The model under review builds one solid part; all positions refer to its coordinate system, in mm. A direction names the side the tool comes from. Coordinates: 2 decimals unless noted, no trailing zeros. Loops run counter-clockwise (first coordinate to the right, second up) from the corner with the lowest first, then second, coordinate; pieces in that order, holes last. Notation, with made-up numbers: M 33,44.5 L 41,44.5 A22 ccw 41,73.5 Z; hole C -5,83.25 d6. An arc over 180 degrees is marked long. Use CSV: the item, a comma, the result in double quotes. Start each with the question number.
1. Tool access review of faces 1 (the flat face through (-16, 6, 29.5)), 2 (the flat face through (-0.14, 3.72, -30.36)), 3 (the flat face through (-0.1, 8.5, 31)), 4 (the flat face through (21.25, 2, 0)), 5 (the flat face through (-21.25, 7, 0)): name each direction out of +Z, -Z, +X, -X, +Y, -Y from which nothing blocks a thin tool from reaching the whole face with its end or side.
2. Add section C-C, the plane x = -14.5. Write out the cut boundary in (y, z), then the cut area to 3 significant figures.
3. Add section B-B, the plane y = 5.25. Write out the cut boundary in (x, z), then the cut area to 3 significant figures.
4. Clearance check with flat-ended pins moving along their axes: P1, Ø2, axis at x = -4.5, y = 7, coming from the -Z side; P2, Ø5, axis at x = 13.5, y = 6.5, coming from the -Z side; P3, Ø0.5, axis at y = 7, z = -30, coming from the -X side. State where each tip first meets the part, or that it passes through.
5. Add section D-D, the plane z = -8.5. Write out the cut boundary in (x, y).
6. Draft analysis for pull direction Y (two halves, no side actions). For faces 6 (the flat face through (0, 0, 0)), 7 (the flat face through (10, 5, -30)), 8 (the flat face through (0, 1, -32.5)), state which applies: +Y half, -Y half, draft (parallel to the pull), parting line (faces both ways), or undercut.
7. For L1, parallel to Y at x = -1, z = 7; L2, parallel to Z at x = 19, y = 7; L3, parallel to X at y = 8.5, z = -30, list the stretches that pass through material, from the lowest coordinate up.
8. Add section A-A, the plane x = 7.5. Write out the cut boundary in (y, z), then the cut area to 3 significant figures.
from build123d import *

# Parameters (mm, degrees)
SKETCH1_W            = 46.5
SKETCH1_H            = 65
BOSS_EXTRUDE1_DEPTH  = 1.5
FILLET1_R            = 3
SKETCH2_W            = 20
SKETCH2_H            = 1.5
BOSS_EXTRUDE2_DEPTH  = 8
CUT_EXTRUDE1_DEPTH   = 24
BOSS_EXTRUDE5_DEPTH  = 20
FILLET4_R            = 0.5
FILLET4_OF_MIRROR1_R = 0.5
BOSS_EXTRUDE6_DEPTH  = 1.5
BOSS_EXTRUDE7_DEPTH  = 0.5
BOSS_EXTRUDE8_START  = -9
BOSS_EXTRUDE8_DEPTH  = 9


with BuildPart() as part:
    # Sketch1 → Boss-Extrude1 (new body)
    with BuildSketch(Plane(origin=(0, 0, 0), x_dir=(1, 0, 0), z_dir=(0, 1, 0))):
        Rectangle(SKETCH1_W, SKETCH1_H)
    extrude(amount=BOSS_EXTRUDE1_DEPTH)

    # Fillet1
    fillet1_edges = [part.edges().sort_by_distance(p)[0] for p in [
        (23.25, 0.75, 32.5),
        (-23.25, 0.75, 32.5),
        (-23.25, 0.75, -32.5),
        (23.25, 0.75, -32.5),
    ]]
    fillet(fillet1_edges, radius=FILLET1_R)

    # Sketch2 → Boss-Extrude2 (add)
    with BuildSketch(Plane(origin=(0, 1.5, 0), x_dir=(1, 0, 0), z_dir=(0, 1, 0))):
        with Locations((0, 29.75)):
            Rectangle(SKETCH2_W, SKETCH2_H)
    boss_extrude2 = extrude(amount=BOSS_EXTRUDE2_DEPTH)

    # Sketch5 → Cut-Extrude1 (cut)
    with BuildSketch(Plane.ZY.offset(10)):
        Polygon((-30.5, 9.5), (-30.5, 1.5), (-30, 9.5), align=None)
    cut_extrude1 = extrude(amount=-CUT_EXTRUDE1_DEPTH, mode=Mode.SUBTRACT)

    # Sketch6 → Boss-Extrude5 (add)
    with BuildSketch(Plane.ZY.offset(10)):
        Polygon((-29, 9.5), (-30, 9.5), (-32, 7.5), (-32, 6), (-29, 6), align=None)
    boss_extrude5 = extrude(amount=-BOSS_EXTRUDE5_DEPTH)

    # Fillet4
    fillet4_edges = [part.edges().sort_by_distance(p)[0] for p in [
        (0, 1.5, -29),
    ]]
    fillet(fillet4_edges, radius=FILLET4_R)

    # Mirror1: Boss-Extrude2, Cut-Extrude1, Boss-Extrude5 across plane
    add(boss_extrude2.mirror(Plane.XY))
    add(cut_extrude1.mirror(Plane.XY), mode=Mode.SUBTRACT)
    add(boss_extrude5.mirror(Plane.XY))

    # Fillet4 of Mirror1
    fillet4_of_mirror1_edges = [part.edges().sort_by_distance(p)[0] for p in [
        (0, 1.5, 29),
    ]]
    fillet(fillet4_of_mirror1_edges, radius=FILLET4_OF_MIRROR1_R)

    # Sketch7 → Boss-Extrude6 (add)
    with BuildSketch(Plane(origin=(0, 1.5, 0), x_dir=(1, 0, 0), z_dir=(0, 1, 0))):
        with BuildLine():
            Line((-11, 30.5), (-20.25, 30.5))
            ThreePointArc((-20.25, 30.5), (-20.957106781, 30.207106781), (-21.25, 29.5))
            Line((-21.25, 29.5), (-21.25, -29.5))
            ThreePointArc((-21.25, -29.5), (-20.957106781, -30.207106781), (-20.25, -30.5))
            Line((-20.25, -30.5), (-11, -30.5))
            Line((-11, -30.5), (-11, -29.5))
            Line((-11, -29.5), (-20.25, -29.5))
            Line((-20.25, -29.5), (-20.25, 29.5))
            Line((-20.25, 29.5), (-11, 29.5))
            Line((-11, 29.5), (-11, 30.5))
        make_face()
        with BuildLine():
            Line((20.25, -29.5), (20.25, 29.5))
            Line((20.25, 29.5), (11, 29.5))
            Line((11, 29.5), (11, 30.5))
            Line((11, 30.5), (20.25, 30.5))
            ThreePointArc((20.25, 30.5), (20.957106781, 30.207106781), (21.25, 29.5))
            Line((21.25, 29.5), (21.25, -29.5))
            ThreePointArc((21.25, -29.5), (20.957106781, -30.207106781), (20.25, -30.5))
            Line((20.25, -30.5), (11, -30.5))
            Line((11, -30.5), (11, -29.5))
            Line((11, -29.5), (20.25, -29.5))
        make_face()
    extrude(amount=BOSS_EXTRUDE6_DEPTH)



with BuildPart() as body_2:
    # Sketch8 → Boss-Extrude7 (new body)
    with BuildSketch(Plane(origin=(0, 11.5, 0), x_dir=(1, 0, 0), z_dir=(0, 1, 0))):
        with BuildLine():
            Line((-11, -30.5), (11, -30.5))
            Line((11, -30.5), (20.25, -30.5))
            ThreePointArc((20.25, -30.5), (20.957106781, -30.207106781), (21.25, -29.5))
            Line((21.25, -29.5), (21.25, 29.5))
            ThreePointArc((21.25, 29.5), (20.957106781, 30.207106781), (20.25, 30.5))
            Line((20.25, 30.5), (11, 30.5))
            Line((11, 30.5), (-11, 30.5))
            Line((-11, 30.5), (-20.25, 30.5))
            ThreePointArc((-20.25, 30.5), (-20.957106781, 30.207106781), (-21.25, 29.5))
            Line((-21.25, 29.5), (-21.25, -29.5))
            ThreePointArc((-21.25, -29.5), (-20.957106781, -30.207106781), (-20.25, -30.5))
            Line((-20.25, -30.5), (-11, -30.5))
        make_face()
    extrude(amount=BOSS_EXTRUDE7_DEPTH)


with BuildPart() as part_1:
    add(part.part)

    add(body_2.part)  # Boss-Extrude8 merges body 2
    # Sketch9 → Boss-Extrude8 (add)
    with BuildSketch(Plane(origin=(0, 12, 0), x_dir=(1, 0, 0), z_dir=(0, 1, 0)).offset(BOSS_EXTRUDE8_START)):
        with BuildLine():
            Line((11, 29.5), (21.25, 29.5))
            ThreePointArc((21.25, 29.5), (20.957106781, 30.207106781), (20.25, 30.5))
            Line((20.25, 30.5), (11, 30.5))
            Line((11, 30.5), (11, 29.5))
        make_face()
        with BuildLine():
            ThreePointArc((20.25, -30.5), (20.957106781, -30.207106781), (21.25, -29.5))
            Line((21.25, -29.5), (11.5, -29.5))
            Line((11.5, -29.5), (11.5, -30.5))
            Line((11.5, -30.5), (20.25, -30.5))
        make_face()
        with BuildLine():
            Line((-11, 29.5), (-11, 30.5))
            Line((-11, 30.5), (-20.25, 30.5))
            ThreePointArc((-20.25, 30.5), (-20.957106781, 30.207106781), (-21.25, 29.5))
            Line((-21.25, 29.5), (-21.25, -29.5))
            ThreePointArc((-21.25, -29.5), (-20.957106781, -30.207106781), (-20.25, -30.5))
            Line((-20.25, -30.5), (-11, -30.5))
            Line((-11, -30.5), (-11, -29.5))
            Line((-11, -29.5), (-20.25, -29.5))
            Line((-20.25, -29.5), (-20.25, 29.5))
            Line((-20.25, 29.5), (-11, 29.5))
        make_face()
    extrude(amount=BOSS_EXTRUDE8_DEPTH)


solid = part_1.part
Computed:
1,face 1,"none"
1,face 2,"-Z"
1,face 3,"+Z"
1,face 4,"+Z, -Z, +X, +Y"
1,face 5,"+Z, -Z, -X, +Y"
2,outline,"M 0,-32.5 L 1.5,-32.5 L 1.5,-30.5 L 12,-30.5 L 12,30.5 L 1.5,30.5 L 1.5,32.5 L 0,32.5 Z; hole M 1.5,-29.5 L 11.5,-29.5 L 11.5,29.5 L 1.5,29.5 Z"
2,area,"148 mm^2"
3,outline,"M -21.25,-29.5 A1 ccw -20.25,-30.5 L -11,-30.5 L -11,-29.5 L -20.25,-29.5 L -20.25,29.5 L -11,29.5 L -11,30.5 L -20.25,30.5 A1 ccw -21.25,29.5 Z; M -10,-30.27 L 10,-30.27 L 10,-29 L -10,-29 Z; M -10,29 L 10,29 L 10,30.27 L -10,30.27 Z; M 11,-30.5 L 20.25,-30.5 A1 ccw 21.25,-29.5 L 11,-29.5 Z; M 11.5,29.5 L 21.25,29.5 A1 ccw 20.25,30.5 L 11.5,30.5 Z"
3,area,"149 mm^2"
4,P1,"stops at z = -32"
4,P2,"stops at z = -30.5"
4,P3,"stops at x = -21.22"
5,outline,"M -23.25,0 L 23.25,0 L 23.25,1.5 L 21.25,1.5 L 21.25,3 L 20.25,3 L 20.25,1.5 L -20.25,1.5 L -20.25,11.5 L 21.25,11.5 L 21.25,12 L -21.25,12 L -21.25,1.5 L -23.25,1.5 Z"
6,face 6,"-Y half"
6,face 7,"undercut"
6,face 8,"draft"
7,L1,"y = 0 to 1.5, 11.5 to 12"
7,L2,"z = -30.5 to -29.5, 29.5 to 30.5"
7,L3,"x = -21.12 to -11, -10 to 10, 11 to 21.12"
8,outline,"M 0,-32.5 L 1.5,-32.5 L 1.5,-30.5 L 6,-30.22 L 6,-32 L 7.5,-32 L 9.5,-30 L 9.5,-29 L 2,-29 A0.5 cw 1.5,-28.5 L 1.5,28.5 A0.5 cw 2,29 L 9.5,29 L 9.5,30 L 7.5,32 L 6,32 L 6,30.22 L 1.5,30.5 L 1.5,32.5 L 0,32.5 Z; M 11.5,-30.5 L 12,-30.5 L 12,30.5 L 11.5,30.5 Z"
8,area,"157 mm^2"
